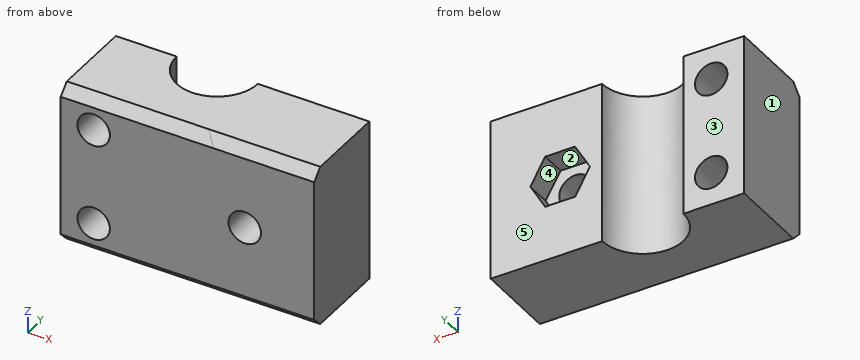
Autodesk Inventor part; units mm, degrees
ref_plane "YZ Plane" through (0, 0, 0) normal (1, 0, 0) x (0, 1, 0)
ref_plane "XZ Plane" through (0, 0, 0) normal (0, 1, 0) x (-1, 0, 0)
ref_plane "XY Plane" through (0, 0, 0) normal (0, 0, 1) x (1, 0, 0)
sketch "Sketch1" plane through (0, 0, 0) normal (0, 1, 0) x (-1, 0, 0)
  line L0 (-50, 16) -> (50, 16)
  line L1 (50, 16) -> (50, -16)
  line L2 (50, -16) -> (-50, -16)
  line L3 (-50, -16) -> (-50, 16)
  point P0 (0, 0)
  point P1 (-50, 0)
  point P2 (0, 16)
  dimension "d0" = 100
  dimension "d1" = 32
extrude "Extrusion1" add sketch "Sketch1" along normal blind 18
sketch "Sketch7" plane through (50, 0, -16) normal (0, 0, -1) x (-1, 0, 0)
  line L0 (100, 0) -> (0, 0)
  line L1 (100, 0) -> (100, 18)
  line L2 (0, 18) -> (100, 18)
  line L3 (0, 0) -> (0, 18)
  circle A0 centre (20, 18) radius 8
  line L4 (100, 18) -> (0, 18)
  circle A1 centre (80, 18) radius 8
  line L5 (20, 18) -> (80, 18) construction
  circle A2 centre (50, 18) radius 5
  point P0 (50, 0)
  dimension "d32" = 60
  dimension "d33" = 16
  dimension "d34" = 10
extrude "Extrusion7" cut sketch "Sketch7" against normal through all contours A1 L2 | L2 A1 | A0 L2 | L2 A0 | A2 L2 | L2 A2
sketch "Sketch8" plane through (50, 0, -16) normal (0, 0, -1) x (-1, 0, 0)
  arc A0 (72, 18) -> (88, 18) centre (80, 18) ccw
  line L0 (55, 18) -> (72, 18)
  arc A1 (45, 18) -> (55, 18) centre (50, 18) ccw
  line L1 (28, 18) -> (45, 18)
  arc A2 (12, 18) -> (28, 18) centre (20, 18) ccw
  line L2 (0, 18) -> (12, 18)
  line L3 (0, 0) -> (0, 18)
  line L4 (100, 0) -> (0, 0)
  line L5 (100, 0) -> (100, 18)
  line L6 (88, 18) -> (100, 18)
  circle A3 centre (50, 18) radius 12
  point P0 (50, 0)
  dimension "d37" = 24
extrude "Extrusion8" cut sketch "Sketch8" against normal blind 9 contours A3 L1 A1 L0 | L0 A1 L1 A3
sketch "Sketch9" plane through (-50, 0, 16) normal (0, 0, 1) x (1, 0, 0)
  arc A0 (12, 18) -> (28, 18) centre (20, 18) ccw
  line L0 (0, 18) -> (12, 18)
  line L1 (0, 0) -> (0, 18)
  line L2 (100, 0) -> (0, 0)
  line L3 (100, 0) -> (100, 18)
  line L4 (88, 18) -> (100, 18)
  arc A1 (72, 18) -> (88, 18) centre (80, 18) ccw
  line L5 (55, 18) -> (72, 18)
  arc A2 (45, 18) -> (55, 18) centre (50, 18) ccw
  line L6 (28, 18) -> (45, 18)
  arc A3 (45, 18) -> (55, 18) centre (50, 18) ccw
  circle A4 centre (50, 18) radius 12.5
  point P0 (50, 18)
  dimension "d49" = 25
extrude "Extrusion9" cut sketch "Sketch9" against normal blind 9 contours A4 L5 A2 L6 | L6 A2 L5 A4
sketch "Sketch11" plane through (0, 0, 0) normal (0, -1, 0) x (1, 0, 0)
  circle A0 centre (43.5, -9.5) radius 3
  circle A1 centre (43.5, 9.5) radius 3
  circle A2 centre (13.7, 0) radius 3
  circle A3 centre (-13.7, 0) radius 3
  circle A4 centre (-43.5, -9.5) radius 3
  circle A5 centre (-43.5, 9.5) radius 3
  circle A6 centre (43.5, 9.5) radius 3.2
  circle A7 centre (43.5, -9.5) radius 3.2
  circle A8 centre (13.7, 0) radius 3.2
  circle A9 centre (-13.7, 0) radius 3.2
  circle A10 centre (-43.5, -9.5) radius 3.2
  circle A11 centre (-43.5, 9.5) radius 3.2
  point P0 (0, 0)
  dimension "d50" = 0.2
extrude "Extrusion10" cut sketch "Sketch11" against normal through all contours A0 | A1 | A2 | A3 | A4 | A5 | A6 | A7 | A8 | A9 | A10 | A11
chamfer "Chamfer3" distance 2 angle 45 2 edges at (0, 0, -16) (0, 0, 16)
sketch "Sketch12" plane through (0, 18, 0) normal (0, 1, 0) x (1, 0, 0)
  circle A0 centre (-13.7, 0) radius 3.2
  circle A1 centre (13.7, 0) radius 3.2
  line L0 (10.7555, 5.1) -> (16.6445, 5.1)
  line L1 (16.6445, 5.1) -> (19.589, 0)
  line L2 (19.589, 0) -> (16.6445, -5.1)
  line L3 (16.6445, -5.1) -> (10.7555, -5.1)
  line L4 (10.7555, -5.1) -> (7.811, 0)
  line L5 (7.811, 0) -> (10.7555, 5.1)
  circle A2 centre (-13.7, 0) radius 3.2
  line L6 (-10.7555, -5.1) -> (-16.6445, -5.1)
  line L7 (-16.6445, -5.1) -> (-19.589, 0)
  line L8 (-19.589, 0) -> (-16.6445, 5.1)
  line L9 (-16.6445, 5.1) -> (-10.7555, 5.1)
  line L10 (-10.7555, 5.1) -> (-7.811, 0)
  line L11 (-7.811, 0) -> (-10.7555, -5.1)
  point P0 (0, 0)
  dimension "d51" = 10.2
extrude "Extrusion11" cut sketch "Sketch12" against normal blind 5
sketch "Sketch13" plane through (0, 0, 0) normal (0, -1, 0) x (1, 0, 0)
  circle A0 centre (-43.5, 9.5) radius 3.2 construction
  circle A1 centre (-13.7, 0) radius 3.2 construction
  circle A2 centre (43.5, -9.5) radius 3.2 construction
  circle A3 centre (43.5, 9.5) radius 3.2 construction
  circle A4 centre (13.7, 0) radius 3.2 construction
  circle A5 centre (-43.5, -9.5) radius 3.2 construction
  line L0 (-50, 14) -> (50, 14) construction
  line L1 (-50, 14) -> (-50, -14) construction
  line L2 (50, -14) -> (-50, -14) construction
  line L3 (50, -14) -> (50, 14) construction
  line L4 (50, -16) -> (50, -14) construction
  line L5 (50, -14) -> (-50, -14) construction
  line L6 (-50, -14) -> (-50, -16) construction
  line L7 (-50, -16) -> (50, -16) construction
  line L8 (-50, 16) -> (-50, 14) construction
  line L9 (-50, 14) -> (50, 14) construction
  line L10 (50, 14) -> (50, 16) construction
  line L11 (50, 16) -> (-50, 16) construction
  line L12 (50, 16) -> (50, -16)
  line L13 (50, 16) -> (-50, 16)
  line L14 (50, -16) -> (0, -16)
  line L15 (0, -16) -> (0, 16)
  line L16 (0, 16) -> (50, 16)
  line L17 (50, 16) -> (50, -16)
  point P0 (0, 0)
extrude "Extrusion12" cut sketch "Sketch13" against normal through all
sketch "Sketch14" plane through (0, 18, 0) normal (0, 1, 0) x (1, 0, 0)
  line L0 (0, 7) -> (0, 16) construction
  line L1 (-12, 16) -> (0, 16) construction
  line L2 (-12, 7) -> (-12, 16) construction
  line L3 (-12, 7) -> (0, 7) construction
  line L4 (0, -16) -> (0, -7) construction
  line L5 (0, -7) -> (-12.5, -7) construction
  line L6 (-12.5, -16) -> (-12.5, -7) construction
  line L7 (0, -16) -> (-12.5, -16) construction
  line L8 (0, -7) -> (0, 7) construction
  line L9 (0, 7) -> (-5, 7) construction
  line L10 (-5, -7) -> (-5, 7) construction
  line L11 (-5, -7) -> (0, -7) construction
  line L12 (-7.811, 0) -> (-10.7555, -5.1) construction
  line L13 (-10.7555, -5.1) -> (-16.6445, -5.1) construction
  line L14 (-16.6445, -5.1) -> (-19.589, 0) construction
  line L15 (-19.589, 0) -> (-16.6445, 5.1) construction
  line L16 (-16.6445, 5.1) -> (-10.7555, 5.1) construction
  line L17 (-10.7555, 5.1) -> (-7.811, 0) construction
  line L18 (-12.5, -7) -> (-5, -7) construction
  line L19 (-5, -7) -> (-5, 7) construction
  line L20 (-5, 7) -> (-12, 7) construction
  line L21 (-12, 7) -> (-12, 16) construction
  line L22 (-12, 16) -> (-22, 16) construction
  line L23 (-22, 16) -> (-22, -16) construction
  line L24 (-22, -16) -> (-12.5, -16) construction
  line L25 (-12.5, -16) -> (-12.5, -7) construction
  line L26 (-5, 7) -> (-12, 7)
  line L27 (-22, 16) -> (-12, 7)
  line L28 (-12, 7) -> (-5, 7)
  line L29 (-5, 7) -> (-5, -7)
  line L30 (0, -7) -> (-12.5, -7)
  line L31 (-22, -16) -> (-38, -16)
  line L32 (-12.5, -7) -> (-22, -16)
  line L33 (0, -16) -> (-12.5, -16)
  line L34 (-22, -16) -> (0, -16)
  line L35 (0, 16) -> (0, 14)
  line L36 (0, -16) -> (0, 16)
  line L37 (-12, 16) -> (-22, 16)
  line L38 (0, 16) -> (-22, 16)
  point P0 (0, 0)
extrude "Extrusion13" add sketch "Sketch14" against normal up to surface (18 mm away)
chamfer "Chamfer4" distance 2 angle 45 2 edges at (-11, 0, 16) (-11, 0, -16)
properties part number "AXBv2" material "PC/ABS Plastic"
Read the model definition and answer for the solid it produces. Units are mm, in the model's axes. Face numbers are marked on the shaded views. A direction names the side the tool comes from. Give positions to 0.01 mm unless a question says otherwise; leave off trailing zeros. Write each loop counter-clockwise with the first axis right and the second up, starting at its lowest first coordinate (ties: lowest second). Pieces come first, ordered by that corner, then holes. Notation, with made-up numbers: (14, 66.5) -> (30, 66.5) arc R14 cw to (30, 89.5) -> close; hole circle Ø11 at (21.25, 27.25). An arc over 180 degrees is marked (long way). Answer as a JSON object with one key per item and string values.
1) Section A-A on x = -43.5 is taken. Write down the section's boundary in (y, z).
Findings below:
{"outline": "(0, -14) -> (2, -16) -> (18, -16) -> (18, -12.7) -> (0, -12.7) -> close; (0, -6.3) -> (18, -6.3) -> (18, 6.3) -> (0, 6.3) -> close; (0, 12.7) -> (18, 12.7) -> (18, 16) -> (2, 16) -> (0, 14) -> close"}
2) Section D-D on y = 6 is taken. Write down the section's boundary in (x, z).
Findings below:
{"outline": "(-50, -16) -> (0, -16) -> (0, 16) -> (-50, 16) -> close; hole circle Ø6.4 at (-43.5, -9.5); hole circle Ø6.4 at (-43.5, 9.5); hole circle Ø6.4 at (-13.7, 0)"}
3) Section B-B on x = -13.7 is taken. Write down the section's boundary in (y, z).
Findings below:
{"outline": "(0, -14) -> (2, -16) -> (18, -16) -> (18, -5.1) -> (13, -5.1) -> (13, -3.2) -> (0, -3.2) -> close; (0, 3.2) -> (13, 3.2) -> (13, 5.1) -> (18, 5.1) -> (18, 16) -> (2, 16) -> (0, 14) -> close"}
4) Section C-C on z = -9.5 is taken. Write down the section's boundary in (x, y).
Findings below:
{"outline": "(-50, 0) -> (-46.7, 0) -> (-46.7, 18) -> (-50, 18) -> close; (-40.3, 0) -> (0, 0) -> (0, 18) -> (-22, 18) arc R8 cw to (-38, 18) -> (-40.3, 18) -> close"}
5) For a pull along X with two mould halves and no side action, classify the marked faces 1, 2 and 3 as pulls with the +X half, pulls with the -X half, needs draft (parallel to the pull), parting line crosses it, or undercut.
Findings below:
{"face 1": "pulls with the -X half", "face 2": "undercut", "face 3": "needs draft"}
6) Straight lines are drawn through the part: probe 1 along Z at (x, y) = (-43.5, 7); probe 2 along X at (y, z) = (15.5, 0.5); probe 3 along Z at (x, y) = (-42, 14.25). For each, find the intervals that lie inside material, in ascending order. Write a range as from..to.
Findings below:
{"probe 1": "z = -16..-12.7, -6.3..6.3, 12.7..16", "probe 2": "x = -50..-37.6, -22.4..-19.3, -8.1..0", "probe 3": "z = -16..-12.33, -6.67..6.67, 12.33..16"}
7) A tool of negligible diameter and unlimited length cuts with its end or side. For the marked faces 4 and 5, from which of +Z, -Z, +X, -X, +Y, -Y can it reach the whole face along a straight path? Write none if from no direction.
Findings below:
{"face 4": "+Y", "face 5": "+Z, -Z, +X, -X, +Y"}
8) Flat-ended cylindrical pins translate along their axes: pin 1 Ø1.5 at (x, z) = (-36, -8.5) entering from +Y; pin 2 Ø8 at (x, z) = (-12, 2.5) entering from +Y. Find the tip coordinate at first contact, or state that the pin passes through.
Findings below:
{"pin 1": "stops at y = 13.71", "pin 2": "stops at y = 18"}
